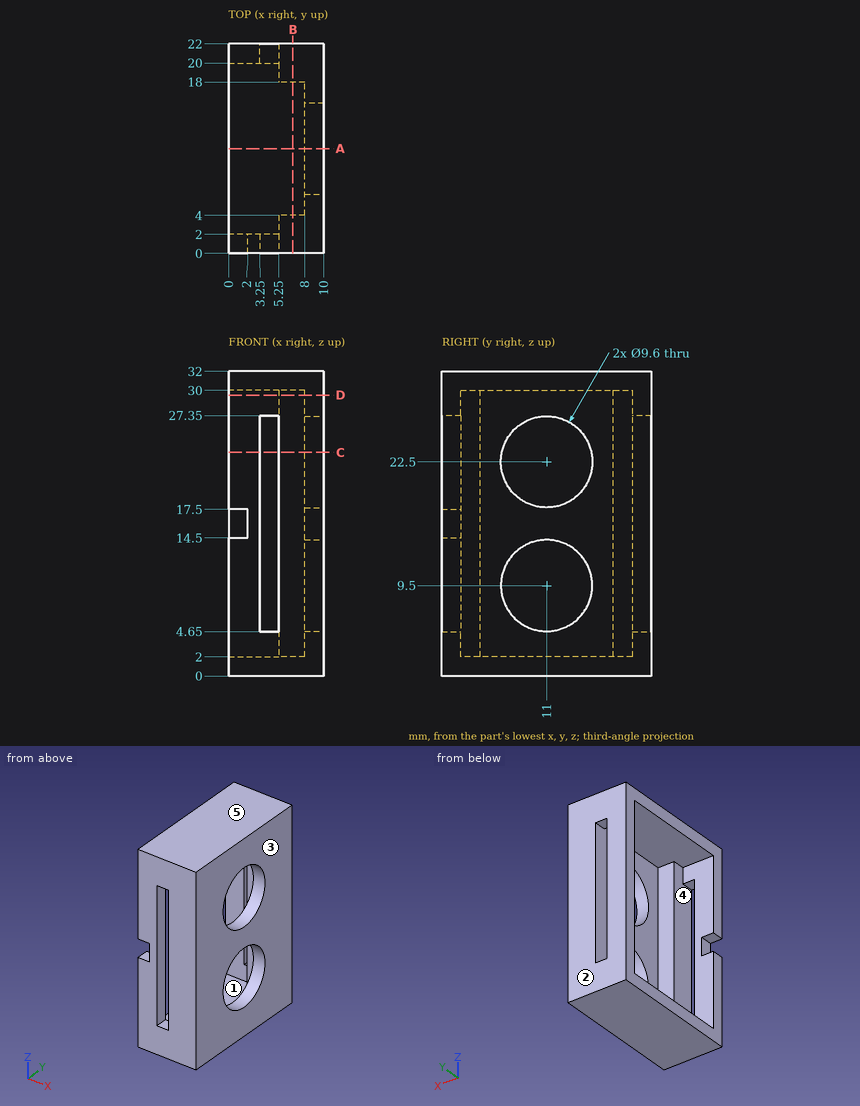
Study the drawing (mm; zero at the part's minimum x, y, z) and answer. A direction names the side the tool comes from. Coordinates: 2 decimals unless noted, no trailing zeros. Loops run counter-clockwise (first coordinate to the right, second up) from the corner with the lowest first, then second, coordinate; pieces in that order, holes last. Notation, with made-up numbers: (86.5, -24.75) -> (108.5, -24.75) arc R23 ccw to (108.5, 10.25) -> close; hole circle Ø6 at (-40, 48.5). An arc over 180 degrees is marked (long way). Write item = value, one per line. Start each with the question number.
1) Find the intervals of material crossed by L1, parallel to Z at x = 9.25, y = 11; L2, parallel to Z at x = 2, y = 19.25; L3, parallel to Y at x = 9, z = 22.5, in increasing order. Write a range as from..to.
2) For the marked faces 1 and 2, determine the directions among +Z, -Z, +X, -X, +Y, -Y from which every point of the face is accessible in a straight line to the end or side of a thin tool.
3) The part is cut by section A-A, the plane y = 11. Determine the outline of the cut face in (x, z).
4) The mould has two halves that part along Z. Classify the marked faces 3, 4 and 5: pulls with the +Z half, pulls with the -Z half, needs draft (parallel to the pull), parting line crosses it, or undercut.
5) The part is cut by section D-D, the plane z = 29.5. Determine the outline of the cut face in (x, y).
6) The part is cut by section C-C, the plane z = 23.5. State how many separate pieces and enclosed holes the cut face has.
7) Given P1, Ø0.6, axis at y = 0.5, z = 16.5, coming from the -X side; P2, Ø4, axis at y = 8.5, z = 17, coming from the -X side, each flat-ended and moving along its own axis, determine where each tip first touches the part or whether it passes through.
8) The part is cut by section B-B, the plane x = 6.75. Determine the outline of the cut face in (y, z), plus the area to 3 significant figures.
Result:
q1.L1 = 0..4.7, 14.3..17.7, 27.3..32
q1.L2 = 0..2, 30..32
q1.L3 = 0..6.2, 15.8..22
q2.face_1 = -X
q2.face_2 = +Z, -Z, +X, -X, +Y
q3.outline = (0, 0) -> (10, 0) -> (10, 4.7) -> (8, 4.7) -> (8, 2) -> (0, 2) -> close; (0, 30) -> (8, 30) -> (8, 27.3) -> (10, 27.3) -> (10, 32) -> (0, 32) -> close; (8, 14.3) -> (10, 14.3) -> (10, 17.7) -> (8, 17.7) -> close
q4.face_3 = needs draft
q4.face_4 = undercut
q4.face_5 = pulls with the +Z half
q5.outline = (0, 0) -> (10, 0) -> (10, 22) -> (0, 22) -> (0, 20) -> (5.25, 20) -> (5.25, 18) -> (8, 18) -> (8, 4) -> (5.25, 4) -> (5.25, 2) -> (0, 2) -> close
q6.separate_pieces = 4
q6.enclosed_holes = 0
q7.P1 = 2
q7.P2 = 8
q8.outline = (0, 0) -> (22, 0) -> (22, 32) -> (0, 32) -> close; hole (4, 2) -> (18, 2) -> (18, 30) -> (4, 30) -> close
q8.area = 312 mm²
